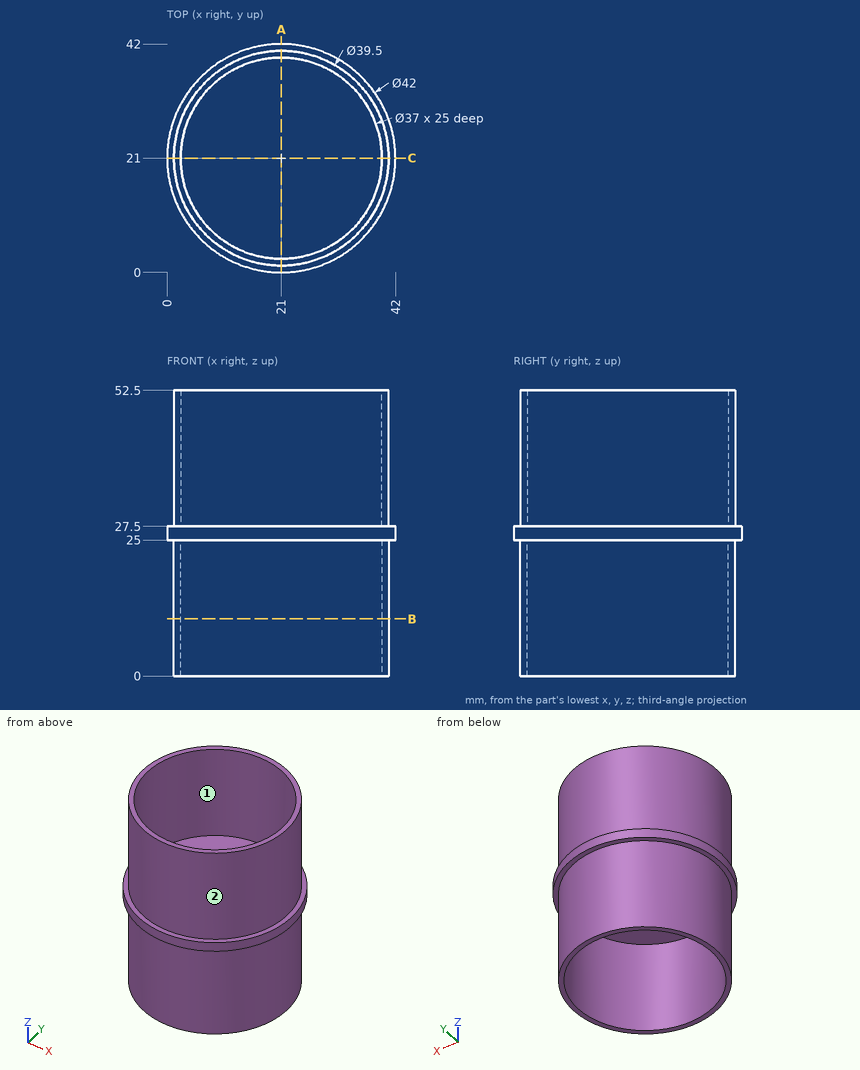
Design review of the part shown in the three views and the two pictorial views. Dimensions are in mm from the part's minimum x, y and z. Round coordinates to 2 decimals unless told otherwise and drop trailing zeros. Loops run counter-clockwise (first coordinate to the right, second up) from the corner with the lowest first, then second, coordinate; pieces in that order, holes last. Notation, with made-up numbers: (3, 11.25) -> (17, 11.25) arc R26 ccw to (17, 46.25) -> close; hole circle Ø2 at (-20, 73). An arc over 180 degrees is marked (long way). Answer as a JSON object with one key per item and string values. Group by question number.
1) For line 1 (Y direction, x = 21, z = 41.5); line 2 (Z direction, x = 23, y = 36), list the stretches that pass through material, from the lowest coordinate up. Write a range as [from, to].
2) We need section A-A on x = 21. Write out the cut boundary in (y, z).
3) For pin 1 Ø6 at (x, y) = (8.5, 32) entering from +Z; pin 2 Ø4 at (x, y) = (24.5, 19) entering from -Z; pin 3 Ø1.5 at (x, z) = (18.5, 38) entering from +Y; pin 4 Ø4 at (y, z) = (32.5, 27.5) entering from -X, all flat-tipped, find the tip position at first contact; note any pin that passes through.
4) Mouldability with a two-part tool opening along Y and no side actions: class the marked faces 1 and 2 as released by +Y, released by -Y, zero draft, split by the parting line, or undercut.
5) We need section B-B on z = 10.5. Write out the cut boundary in (x, y), then the cut area to 3 significant figures.
Result set:
{
 "1": {"line 1": "[1.25, 2.5], [39.5, 40.75]", "line 2": "[25, 27.5]"},
 "2": {"outline": "(0, 25) -> (1.25, 25) -> (1.25, 0) -> (2.5, 0) -> (2.5, 25) -> (39.5, 25) -> (39.5, 0) -> (40.75, 0) -> (40.75, 25) -> (42, 25) -> (42, 27.5) -> (40.75, 27.5) -> (40.75, 52.5) -> (39.5, 52.5) -> (39.5, 27.5) -> (2.5, 27.5) -> (2.5, 52.5) -> (1.25, 52.5) -> (1.25, 27.5) -> (0, 27.5) -> close"},
 "3": {"pin 1": "z = 52.5", "pin 2": "z = 25", "pin 3": "y = 40.67", "pin 4": "x = 2.27"},
 "4": {"face 1": "undercut", "face 2": "split by the parting line"},
 "5": {"outline": "circle Ø39.5 at (21, 21); hole circle Ø37 at (21, 21)", "area": "150 mm²"}
}
